```python
from build123d import *

# Parameters (mm, degrees)
F0_W      = 20
F0_H      = 20
F1_DEPTH  = 20
F2_W      = 5
F2_H      = 5
F3_DEPTH  = 15
F4_R      = 2.1
F5_DEPTH  = 25
F6_W      = 5
F6_H      = 5
F7_DEPTH  = 15
F8_R      = 2.1
F9_DEPTH  = 25
F10_W     = 5
F10_H     = 5
F11_DEPTH = 15
F12_R     = 2.1
F13_DEPTH = 25
F14_R     = 1


with BuildPart() as f1:
    # F0 (on Front) → F1 (new body)
    with BuildSketch(Plane.XZ):
        with Locations((10, 10)):
            Rectangle(F0_W, F0_H)
    extrude(amount=F1_DEPTH)

    # F2 (on face) → F3 (cut)
    with BuildSketch(Plane.XZ.offset(20)):
        with Locations((7.5, 12.5)):
            Rectangle(F2_W, F2_H)
        with Locations((12.5, 12.5)):
            Rectangle(F2_W, F2_H)
        with Locations((12.5, 7.5)):
            Rectangle(F2_W, F2_H)
        with Locations((7.5, 7.5)):
            Rectangle(F2_W, F2_H)
    extrude(amount=-F3_DEPTH, mode=Mode.SUBTRACT)

    # F4 (on face) → F5 (cut)
    with BuildSketch(Plane.XZ.offset(5)):
        with Locations((10, 10)):
            Circle(F4_R)
    extrude(amount=-F5_DEPTH, mode=Mode.SUBTRACT)

    # F6 (on face) → F7 (cut)
    with BuildSketch(Plane.XY.offset(20)):
        with Locations((7.5, -7.5)):
            Rectangle(F6_W, F6_H)
        with Locations((12.5, -7.5)):
            Rectangle(F6_W, F6_H)
        with Locations((12.5, -12.5)):
            Rectangle(F6_W, F6_H)
        with Locations((7.5, -12.5)):
            Rectangle(F6_W, F6_H)
    extrude(amount=-F7_DEPTH, mode=Mode.SUBTRACT)

    # F8 (on face) → F9 (cut)
    with BuildSketch(Plane.XY.offset(5)):
        with Locations((10, -10)):
            Circle(F8_R)
    extrude(amount=-F9_DEPTH, mode=Mode.SUBTRACT)

    # F10 (on face) → F11 (cut)
    with BuildSketch(Plane.YZ.offset(20)):
        with Locations((-12.5, 12.5)):
            Rectangle(F10_W, F10_H)
        with Locations((-7.5, 12.5)):
            Rectangle(F10_W, F10_H)
        with Locations((-7.5, 7.5)):
            Rectangle(F10_W, F10_H)
        with Locations((-12.5, 7.5)):
            Rectangle(F10_W, F10_H)
    extrude(amount=-F11_DEPTH, mode=Mode.SUBTRACT)

    # F12 (on face) → F13 (cut)
    with BuildSketch(Plane.YZ.offset(5)):
        with Locations((-10, 10)):
            Circle(F12_R)
    extrude(amount=-F13_DEPTH, mode=Mode.SUBTRACT)

    # F14
    f14_edges = [f1.edges().sort_by_distance(p)[0] for p in [
        (20, -10, 20),
        (10, -20, 20),
        (20, -20, 10),
    ]]
    fillet(f14_edges, radius=F14_R)


solid = f1.part
```
Input: part model. Units: mm. Frame: model coordinates. A direction names the side the tool comes from. Coordinates: 2 decimals unless noted, no trailing zeros. Write each loop counter-clockwise with the first axis right and the second up, starting at its lowest first coordinate (ties: lowest second). Pieces come first, ordered by that corner, then holes. Notation, with made-up numbers: (60.5, 54.25) -> (105.5, 54.25) arc R13 ccw to (105.5, 59.25) -> close; hole circle Ø11 at (36.5, 76). An arc over 180 degrees is marked (long way). Answer as a JSON object with one key per item and string values.
1. Access query for faces 4 (the face through (15, -18, 10)), 5 (the face through (10, -15, 18)), 6 (the face through (18, -15, 10)), 7 (the face through (5, -12, 13)), 8 (the face through (0, -7.6, 9.9)). Directions: +Z, -Z, +X, -X, +Y, -Y. A direction counts if a zero-diameter tool reaches every point of the face in a straight line with its end or side. Return the directions, or none.
Result set:
{"face 4": "-Y", "face 5": "+Z", "face 6": "+X", "face 7": "none", "face 8": "+Z, -Z, -X, +Y, -Y"}
2. Material intervals for line 1 (Z direction, x = 1.4, y = -10); line 2 (Y direction, x = 17.5, z = 13); line 3 (X direction, y = -18.75, z = 13.5), sorted ascending. Write a range as from..to.
Result set:
{"line 1": "z = 0..7.9, 12.1..20", "line 2": "y = -20..-15, -5..0", "line 3": "x = 0..5, 15..20"}
3. Section C-C on y = -5.75. Return the cut outline in (x, z), then the cut area to 3 significant figures.
Result set:
{"outline": "(0, 0) -> (20, 0) -> (20, 5) -> (5, 5) -> (5, 20) -> (0, 20) -> close; (15, 15) -> (20, 15) -> (20, 19) arc R1 ccw to (19, 20) -> (15, 20) -> close", "area": "200 mm2"}
4. Mould query, pull axis Z, two halves, no side actions, for faces 1 (the face through (19.699, -9.633, 19.715)), 2 (the face through (18, -10, 15)), 3 (the face through (19.699, -19.715, 9.633)). Classes: released by +Z, released by -Z, zero draft, split by the parting line, or undercut.
Result set:
{"face 1": "released by +Z", "face 2": "undercut", "face 3": "zero draft"}
5. Section B-B on x = 18. Return the cut outline in (y, z), then the cut area to 3 significant figures.
Result set:
{"outline": "(-20, 0) -> (0, 0) -> (0, 20) -> (-19, 20) arc R1 ccw to (-20, 19) -> close; hole (-15, 5) -> (-5, 5) -> (-5, 15) -> (-15, 15) -> close", "area": "300 mm2"}
6. First-contact query: P1, Ø2.5, axis at x = 10, z = 10, coming from the -Y side; P2, Ø4.5, axis at x = 12.5, y = -12, coming from the +Z side. Flat tips, straight axial feed; report the tip coordinate or a pass-through.
Result set:
{"P1": "passes through", "P2": "stops at z = 5"}
7. Section D-D on z = 5.5. Return the cut outline in (x, y).
Result set:
{"outline": "(0, -20) -> (5, -20) -> (5, -5) -> (20, -5) -> (20, 0) -> (0, 0) -> close; (15, -20) -> (19, -20) arc R1 ccw to (20, -19) -> (20, -15) -> (15, -15) -> close"}
8. Section A-A on y = -10. Return the cut outline in (x, z).
Result set:
{"outline": "(0, 0) -> (7.9, 0) -> (7.9, 5) -> (5, 5) -> (5, 7.9) -> (0, 7.9) -> close; (0, 12.1) -> (5, 12.1) -> (5, 20) -> (0, 20) -> close; (12.1, 0) -> (20, 0) -> (20, 5) -> (12.1, 5) -> close; (15, 15) -> (20, 15) -> (20, 19) arc R1 ccw to (19, 20) -> (15, 20) -> close"}
